Work out the finished part from the listing and answer in its coordinate system (mm). Face numbers are marked on the shaded views. Give positions to 0.01 mm unless a question says otherwise; leave off trailing zeros. Loops run counter-clockwise (first coordinate to the right, second up) from the corner with the lowest first, then second, coordinate; pieces in that order, holes last. Notation, with made-up numbers: M -38.75,81.25 L -3.75,81.25 A10 ccw -3.75,100.25 Z; hole C -18,-24 d3. An arc over 180 degrees is marked long. Answer as a JSON object with one key per item and string values. Group by question number.
```python
from build123d import *

# Parameters (mm, degrees)
SKETCH_1_R             = 8.75
EXTRUDE_1_DEPTH        = 5
HOLE_WIZARD_M3_1_D     = 2.5
HOLE_WIZARD_M3_1_DEPTH = 5
SKETCH_4_R             = 1.5
CUT_EXTRUDE_1_DEPTH    = 6


with BuildPart() as part:
    # 스케치1 → 보스-돌출1 (new body)
    with BuildSketch(Plane.XY):
        Circle(SKETCH_1_R)
    extrude(amount=EXTRUDE_1_DEPTH)

    # M3 나사 구멍1
    with Locations(Plane.XY.offset(5)):
        with Locations((0, 6.35), (6.35, 0), (0, -6.35), (-6.35, 0)):
            Hole(HOLE_WIZARD_M3_1_D / 2, depth=HOLE_WIZARD_M3_1_DEPTH)

    # 스케치4 → 컷-돌출1 (cut, through all)
    with BuildSketch(Plane.XY.offset(5)):
        Circle(SKETCH_4_R)
    extrude(amount=-CUT_EXTRUDE_1_DEPTH, mode=Mode.SUBTRACT)


solid = part.part
```
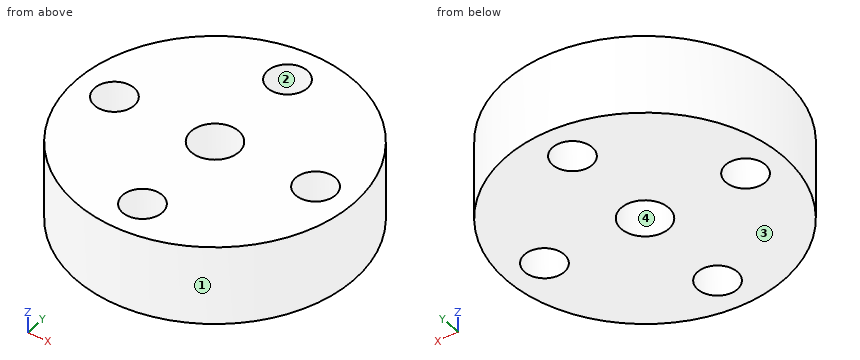
Item 1: Find the intervals of material crossed by probe 1 along Y at (x, z) = (0, 2.8); probe 2 along X at (y, z) = (1, 2.65); probe 3 along Y at (x, z) = (6.5, 4), in increasing order. Write a range as [from, to].
Item 2: Given pin 1 Ø1.5 at (x, z) = (4.5, 1) entering from +Y; pin 2 Ø3 at (x, y) = (6.35, 0) entering from +Z, each flat-ended and moving along its own axis, determine where each tip first touches the part or whether it passes through.
Item 3: For a pull along Y with two mould halves and no side action, classify the marked faces 1, 2, 3 and 4 as pulls with the +Y half, pulls with the -Y half, needs draft (parallel to the pull), parting line crosses it, or undercut.
Item 4: A cutting plane is placed at B-B (x = -7). Determine the outline of the cut face in (y, z), and give its area (3 significant figures).
Item 5: A cutting plane is placed at D-D (z = 1.5). Determine the outline of the cut face in (x, y).
Item 6: A cutting plane is placed at A-A (x = 0). Determine the outline of the cut face in (y, z).
Item 7: A cutting plane is placed at C-C (y = -6.35). Determine the outline of the cut face in (x, z), and give its area (3 significant figures).
The answers:
{
 "1": {"probe 1": "y = [-8.75, -7.6], [-5.1, -1.5], [1.5, 5.1], [7.6, 8.75]", "probe 2": "x = [-8.69, -7.1], [-5.6, -1.12], [1.12, 5.6], [7.1, 8.69]", "probe 3": "y = [-5.86, -1.24], [1.24, 5.86]"},
 "2": {"pin 1": "stops at y = 7.91", "pin 2": "stops at z = 5"},
 "3": {"face 1": "parting line crosses it", "face 2": "undercut", "face 3": "needs draft", "face 4": "undercut"},
 "4": {"outline": "M -5.25,0 L -1.07,0 L -1.07,5 L -5.25,5 Z; M 1.07,0 L 5.25,0 L 5.25,5 L 1.07,5 Z", "area": "41.8 mm^2"},
 "5": {"outline": "C 0,0 d17.5; hole C -6.35,0 d2.5; hole C 0,0 d3; hole C 0,-6.35 d2.5; hole C 0,6.35 d2.5; hole C 6.35,0 d2.5"},
 "6": {"outline": "M -8.75,0 L -7.6,0 L -7.6,5 L -8.75,5 Z; M -5.1,0 L -1.5,0 L -1.5,5 L -5.1,5 Z; M 1.5,0 L 5.1,0 L 5.1,5 L 1.5,5 Z; M 7.6,0 L 8.75,0 L 8.75,5 L 7.6,5 Z"},
 "7": {"outline": "M -6.02,0 L -1.25,0 L -1.25,5 L -6.02,5 Z; M 1.25,0 L 6.02,0 L 6.02,5 L 1.25,5 Z", "area": "47.7 mm^2"}
}
